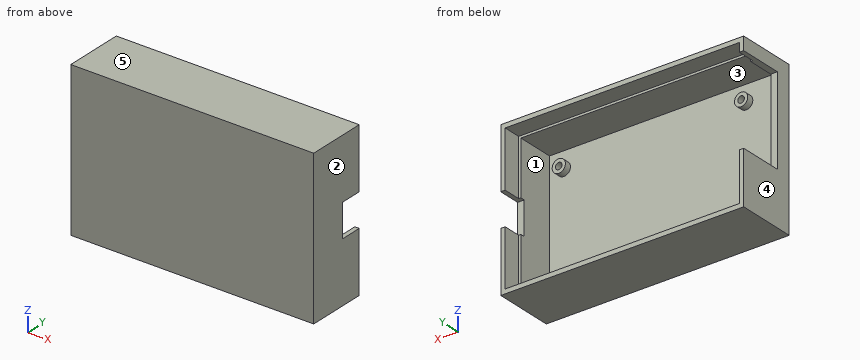
```python
from build123d import *

# Parameters (mm, degrees)
CROQUIS1_W              = 110
CROQUIS1_H              = 70
SALIENTE_EXTRUIR1_DEPTH = 2
CROQUIS2_W              = 110
CROQUIS2_H              = 70
CROQUIS2_W_2            = 104
CROQUIS2_H_2            = 64
SALIENTE_EXTRUIR2_DEPTH = 25
CROQUIS3_W              = 106
CROQUIS3_H              = 66
CORTAR_EXTRUIR1_DEPTH   = 8
CROQUIS4_R              = 3
SALIENTE_EXTRUIR3_DEPTH = 3
CROQUIS6_R              = 1.5
CORTAR_EXTRUIR2_DEPTH   = 4
CROQUIS7_W              = 6
CROQUIS7_H              = 40
CORTAR_EXTRUIR3_DEPTH   = 20
CROQUIS8_W              = 9.353871772
CROQUIS8_H              = 15
CORTAR_EXTRUIR4_DEPTH   = 10


with BuildPart() as part:
    # Croquis1 → Saliente-Extruir1 (new body)
    with BuildSketch(Plane(origin=(0, 0, 0), x_dir=(1, 0, 0), z_dir=(0, 1, 0))):
        Rectangle(CROQUIS1_W, CROQUIS1_H)
    extrude(amount=SALIENTE_EXTRUIR1_DEPTH)

    # Croquis2 → Saliente-Extruir2 (add)
    with BuildSketch(Plane(origin=(0, 2, 0), x_dir=(1, 0, 0), z_dir=(0, 1, 0))):
        Rectangle(CROQUIS2_W, CROQUIS2_H)
        Rectangle(CROQUIS2_W_2, CROQUIS2_H_2, mode=Mode.SUBTRACT)
    extrude(amount=SALIENTE_EXTRUIR2_DEPTH)

    # Croquis3 → Cortar-Extruir1 (cut)
    with BuildSketch(Plane(origin=(0, 27, 0), x_dir=(1, 0, 0), z_dir=(0, 1, 0))):
        Rectangle(CROQUIS3_W, CROQUIS3_H)
    extrude(amount=-CORTAR_EXTRUIR1_DEPTH, mode=Mode.SUBTRACT)

    # Croquis4 → Saliente-Extruir3 (add)
    with BuildSketch(Plane(origin=(0, 2, 0), x_dir=(1, 0, 0), z_dir=(0, 1, 0))):
        with Locations(Location((-37.03, -24.46, 0), (0, 0, 90))):
            Circle(CROQUIS4_R)
        with Locations(Location((-35.76, 23.8, 0), (0, 0, 90))):
            Circle(CROQUIS4_R)
        with Locations(Location((39.17, 23.8, 0), (0, 0, 90))):
            Circle(CROQUIS4_R)
        with Locations(Location((45.52, -24.46, 0), (0, 0, 90))):
            Circle(CROQUIS4_R)
    extrude(amount=SALIENTE_EXTRUIR3_DEPTH)

    # Croquis6 → Cortar-Extruir2 (cut)
    with BuildSketch(Plane(origin=(0, 5, 0), x_dir=(1, 0, 0), z_dir=(0, 1, 0))):
        with Locations(Location((-35.76, 23.8, 0), (0, 0, 270))):
            Circle(CROQUIS6_R)
        with Locations(Location((-37.03, -24.46, 0), (0, 0, 270))):
            Circle(CROQUIS6_R)
        with Locations(Location((39.17, 23.8, 0), (0, 0, 270))):
            Circle(CROQUIS6_R)
        with Locations(Location((45.52, -24.46, 0), (0, 0, 270))):
            Circle(CROQUIS6_R)
    extrude(amount=-CORTAR_EXTRUIR2_DEPTH, mode=Mode.SUBTRACT)

    # Croquis7 → Cortar-Extruir3 (cut)
    with BuildSketch(Plane(origin=(0, 27, 0), x_dir=(1, 0, 0), z_dir=(0, 1, 0))):
        with Locations((-55, -9)):
            Rectangle(CROQUIS7_W, CROQUIS7_H)
    extrude(amount=-CORTAR_EXTRUIR3_DEPTH, mode=Mode.SUBTRACT)

    # Croquis8 → Cortar-Extruir4 (cut)
    with BuildSketch(Plane(origin=(0, 27, 0), x_dir=(1, 0, 0), z_dir=(0, 1, 0))):
        with Locations((53, 0)):
            Rectangle(CROQUIS8_W, CROQUIS8_H)
    extrude(amount=-CORTAR_EXTRUIR4_DEPTH, mode=Mode.SUBTRACT)


solid = part.part
```
Geometry: final body of the model. Coordinates: model frame, mm. Face numbers are marked on the shaded views. A direction names the side the tool comes from. Give positions to 0.01 mm unless a question says otherwise; leave off trailing zeros. Order: outer loops, then holes, each group sorted by start corner. A loop starts at its lowest first (then second) coordinate and runs counter-clockwise, first axis right, second up. Notation, with made-up numbers: (-24, -21.75) -> (33, -21.75) arc R29 cw to (33, 0.25) -> close; hole circle Ø5 at (-17.75, 82.5). An arc over 180 degrees is marked (long way). Write each question's results on one line, items separated by ' | '. Start each with the question number.
1) Section A-A (z = -13). Return loops of the section in (x, y).
2) Line query: line 1 (X direction, y = 1.8, z = -23.8); line 2 (X direction, y = 1.8, z = 24.46); line 3 (X direction, y = 3.35, z = -23.8). Output: solid intervals per line, ascending. Write a range as from..to.
3) Section C-C (z = 24.46). Return loops of the section in (x, y), then the cut area to 3 significant figures.
4) First-contact query: pin 1 (2.5 mm diameter, centred on x = 39.17, z = -23.8, fed in from +Y); pin 2 (9 mm diameter, centred on y = 24.5, z = 19, fed in from -X); pin 3 (3 mm diameter, centred on x = -35, z = -23, fed in from +Y). Flat tips, straight axial feed; report the tip coordinate or a pass-through.
5) Section D-D (x = 39.17). Return loops of the section in (y, z).
6) Section B-B (x = 8.5). Return loops of the section in (y, z), then the cut area to 3 significant figures.
7) Draft query along Z for the marked faces 3, 4 and 5. Return one class per face: pulls with the +Z half, pulls with the -Z half, needs draft (parallel to the pull), parting line crosses it, or undercut.
8) Set-up query: the marked faces 1 and 2. Return all of +Z, -Z, +X, -X, +Y, -Y with unobstructed straight access to the full face (end or side cutting, diameter ignored); none if empty.
Calculated:
1) outline: (-55, 0) -> (55, 0) -> (55, 27) -> (53, 27) -> (53, 19) -> (52, 19) -> (52, 2) -> (-52, 2) -> (-52, 19) -> (-53, 19) -> (-53, 27) -> (-55, 27) -> close
2) line 1: -55..-37.26, -34.26..37.67, 40.67..55 | line 2: -55..-38.53, -35.53..44.02, 47.02..55 | line 3: -55..-52, -38.76..-37.26, -34.26..-32.76, 36.17..37.67, 40.67..42.17, 52..55
3) outline: (-55, 0) -> (55, 0) -> (55, 27) -> (53, 27) -> (53, 19) -> (52, 19) -> (52, 2) -> (48.52, 2) -> (48.52, 5) -> (47.02, 5) -> (47.02, 1) -> (44.02, 1) -> (44.02, 5) -> (42.52, 5) -> (42.52, 2) -> (-34.03, 2) -> (-34.03, 5) -> (-35.53, 5) -> (-35.53, 1) -> (-38.53, 1) -> (-38.53, 5) -> (-40.03, 5) -> (-40.03, 2) -> (-52, 2) -> (-52, 7) -> (-55, 7) -> close | area: 314 mm2
4) pin 1: y = 1 | pin 2: x = 53 | pin 3: y = 5
5) outline: (0, -35) -> (27, -35) -> (27, -33) -> (19, -33) -> (19, -32) -> (2, -32) -> (2, -26.8) -> (5, -26.8) -> (5, -25.3) -> (1, -25.3) -> (1, -22.3) -> (5, -22.3) -> (5, -20.8) -> (2, -20.8) -> (2, 32) -> (19, 32) -> (19, 33) -> (27, 33) -> (27, 35) -> (0, 35) -> close
6) outline: (0, -35) -> (27, -35) -> (27, -33) -> (19, -33) -> (19, -32) -> (2, -32) -> (2, 32) -> (19, 32) -> (19, 33) -> (27, 33) -> (27, 35) -> (0, 35) -> close | area: 274 mm2
7) face 3: undercut | face 4: needs draft | face 5: pulls with the +Z half
8) face 1: +Y | face 2: +Z, -Z, +X, +Y, -Y
